CAD build for the part. Positions are in the model's coordinates, mm. A direction names the side the tool comes from. Coordinates: 2 decimals unless noted, no trailing zeros. Order: outer loops, then holes, each group sorted by start corner. A loop starts at its lowest first (then second) coordinate and runs counter-clockwise, first axis right, second up. Notation, with made-up numbers: M 32.5,84.5 L 72.5,84.5 A35 ccw 72.5,118.5 Z; hole C 72,-25 d7. An arc over 180 degrees is marked long. Write item = value, one per line.
from build123d import *

# Parameters (mm, degrees)
SKETCH5_OUTSIDE_W   = 26.73
SKETCH5_OUTSIDE_H   = 26.73
CUT_EXTRUDE1_DEPTH  = 10
BOSS_EXTRUDE3_DEPTH = 0.24


with BuildPart() as part:
    # Sketch3 → Revolve1 (revolve)
    with BuildSketch(Plane(origin=(0, 0, 0), x_dir=(0, 0, -1), z_dir=(1, 0, 0))):
        with BuildLine():
            Line((-2, 5), (-2, 9))
            Line((-2, 9), (0, 9))
            Line((0, 9), (0, 7.5))
            Line((0, 7.5), (0, 7.26))
            Line((0, 7.26), (0.24, 7.26))
            Line((0.24, 7.26), (0.24, 7.5))
            Line((0.24, 7.5), (10.787867966, 7.5))
            Line((10.787867966, 7.5), (11, 7.287867966))
            Line((11, 7.287867966), (11, 0))
            Line((11, 0), (-11, 0))
            ThreePointArc((-11, 0), (-9.535533906, 3.535533906), (-6, 5))
            Line((-6, 5), (-2.24, 5))
            Line((-2.24, 5), (-2.24, 4.76))
            Line((-2.24, 4.76), (-2, 4.76))
            Line((-2, 4.76), (-2, 5))
        make_face()
    revolve(axis=Axis((0, 0, 11), (0, 0, -1)))

    # Sketch5 outside → Cut-Extrude1 (cut, through all)
    with BuildSketch(Plane.XY.offset(2)):
        Rectangle(SKETCH5_OUTSIDE_W, SKETCH5_OUTSIDE_H)
        with BuildLine():
            Line((-5, 0), (-2.5, -4.330127019))
            ThreePointArc((-2.5, -4.330127019), (0, -5), (2.5, -4.330127019))
            Line((2.5, -4.330127019), (5, 0))
            Line((5, 0), (2.5, 4.330127019))
            ThreePointArc((2.5, 4.330127019), (0, 5), (-2.5, 4.330127019))
            Line((-2.5, 4.330127019), (-5, 0))
        make_face(mode=Mode.SUBTRACT)
    extrude(amount=CUT_EXTRUDE1_DEPTH, mode=Mode.SUBTRACT)

    # Sketch7 → Boss-Extrude3 (add)
    with BuildSketch(Plane.XY.offset(2)):
        with BuildLine():
            Line((-4.738382517, -0.453134773), (-5, 0))
            Line((-5, 0), (-4.738382517, 0.453134773))
            ThreePointArc((-4.738382517, 0.453134773), (-4.76, 0), (-4.738382517, -0.453134773))
        make_face()
        with BuildLine():
            Line((4.738382517, 0.453134773), (5, 0))
            Line((5, 0), (4.738382517, -0.453134773))
            ThreePointArc((4.738382517, -0.453134773), (4.76, 0), (4.738382517, 0.453134773))
        make_face()
    extrude(amount=BOSS_EXTRUDE3_DEPTH)


solid = part.part
(1) Slice it at B-B, the plane z = 3. Write the cut outline in (x, y), then the cut area to 3 significant figures.
Evaluation:
outline = M -5,0 L -2.5,-4.33 A5 ccw 2.5,-4.33 L 5,0 L 2.5,4.33 A5 ccw -2.5,4.33 Z
area = 69.5 mm²
(2) Slice it at A-A, the plane x = 0. Write the cut outline in (y, z).
Evaluation:
outline = M -9,0 L -7.26,0 L -7.26,-0.24 L -7.5,-0.24 L -7.5,-10.79 L -7.29,-11 L 7.29,-11 L 7.5,-10.79 L 7.5,-0.24 L 7.26,-0.24 L 7.26,0 L 9,0 L 9,2 L 4.76,2 L 4.76,2.24 L 5,2.24 L 5,6 A5 ccw -5,6 L -5,2.24 L -4.76,2.24 L -4.76,2 L -9,2 Z
(3) Tool access for faces 1 (the face through (0.33, -7.493, -5.588)), 2 (the face through (7.4, 0.6, 0)), 3 (the face through (0, -5, 4)): list every direction of +Z, -Z, +X, -X, +Y, -Y with a clear straight run to the whole face (end or side of a thin tool).
Evaluation:
face_1 = -Z
face_2 = none
face_3 = +Z, -Y
(4) Slice it at D-D, the plane z = 9. Write the cut outline in (x, y).
Evaluation:
outline = C 0,0 d8
(5) Slice it at C-C, the plane z = -4.5. Write the cut outline in (x, y).
Evaluation:
outline = C 0,0 d15
(6) Pin check, flat tips, straight feed: pin 1 Ø6 at (y, z) = (6.5, 5.5) entering from -X; pin 2 Ø4 at (y, z) = (6, 4.5) entering from +X; pin 3 Ø5 at (x, z) = (-1, 5) entering from -Y; pin 4 Ø9 at (x, y) = (-2, 0.5) entering from +Z. Stop position of each tip, or through.
Evaluation:
pin_1 = -2.98
pin_2 = 2.69
pin_3 = -5
pin_4 = 11
(7) Wall check: line 1 (Z direction, x = -6.25, y = -4.25); line 2 (Z direction, x = 2.25, y = 6.25); line 3 (Y direction, x = -0.75, z = -8.25). Give the ranges that are in metal, low to high. Write a range as from..to.
Evaluation:
line_1 = 0..2
line_2 = -11..2
line_3 = -7.46..7.46
